```python
from build123d import *

# Parameters (mm, degrees)
SALIENTE_EXTRUIR1_DEPTH = 50.8
CROQUIS2_R              = 6.5
CORTAR_EXTRUIR1_DEPTH   = 10
CROQUIS3_R              = 6.5
CORTAR_EXTRUIR2_DEPTH   = 10
CROQUIS4_W              = 50.8
CROQUIS4_H              = 74.5
CORTAR_EXTRUIR3_DEPTH   = 10
CROQUIS5_R              = 6.35
CORTAR_EXTRUIR4_DEPTH   = 10


with BuildPart() as part:
    # Croquis1 → Saliente-Extruir1 (new body)
    with BuildSketch(Plane(origin=(0, 0, 0), x_dir=(0, 0, -1), z_dir=(1, 0, 0))):
        Polygon((-6.31, 95.93), (0, 95.93), (0, 0), (-902.2, 0), (-902.2, 6.31), (-6.31, 6.31), align=None)
    extrude(amount=SALIENTE_EXTRUIR1_DEPTH)

    # Croquis2 → Cortar-Extruir1 (cut)
    with BuildSketch(Plane(origin=(0, 0, 0), x_dir=(-1, 0, 0), z_dir=(0, -1, 0))):
        with Locations(Location((-25.4, -885.7, 0), (0, 0, 90))):
            Circle(CROQUIS2_R)
        with Locations(Location((-25.4, -854.7, 0), (0, 0, 90))):
            Circle(CROQUIS2_R)
    extrude(amount=-CORTAR_EXTRUIR1_DEPTH, mode=Mode.SUBTRACT)

    # Croquis3 → Cortar-Extruir2 (cut)
    with BuildSketch(Plane(origin=(0, 0, 0), x_dir=(-1, 0, 0), z_dir=(0, 0, -1))):
        with Locations(Location((-25.4, 70.53, 0), (0, 0, 90))):
            Circle(CROQUIS3_R)
    extrude(amount=-CORTAR_EXTRUIR2_DEPTH, mode=Mode.SUBTRACT)

    # Croquis4 → Cortar-Extruir3 (cut)
    with BuildSketch(Plane.XZ):
        with Locations((25.4, 864.95)):
            Rectangle(CROQUIS4_W, CROQUIS4_H)
    extrude(amount=-CORTAR_EXTRUIR3_DEPTH, mode=Mode.SUBTRACT)

    # Croquis5 → Cortar-Extruir4 (cut)
    with BuildSketch(Plane(origin=(0, 0, 0), x_dir=(-1, 0, 0), z_dir=(0, -1, 0))):
        with Locations(Location((-25.4, -765.81, 0), (0, 0, 90))):
            Circle(CROQUIS5_R)
        with Locations(Location((-25.4, -805.81, 0), (0, 0, 90))):
            Circle(CROQUIS5_R)
    extrude(amount=-CORTAR_EXTRUIR4_DEPTH, mode=Mode.SUBTRACT)


solid = part.part
```
Input: part model. Units: mm. Frame: model coordinates. A direction names the side the tool comes from. Give positions to 0.01 mm unless a question says otherwise; leave off trailing zeros. Order: outer loops, then holes, each group sorted by start corner. A loop starts at its lowest first (then second) coordinate and runs counter-clockwise, first axis right, second up. Notation, with made-up numbers: M 30,-28 L 68,-28 A20 cw 68,-11 Z; hole C 37,56.25 d1. An arc over 180 degrees is marked long. One line per question, with ' | ' between items. Start each with the question number.
1. Material intervals for probe 1 along X at (y, z) = (1, 805); probe 2 along X at (y, z) = (70.53, 1.5); probe 3 along Z at (x, y) = (20.5, 18.5), sorted ascending. Write a range as [from, to].
2. Pull-direction query (Y, two-part tool) for faces 1 (the face through (25, 0, 408)), 2 (the face through (25.679, 3.111, 772.154)), 3 (the face through (21.445, 65.372, 3.111)); classes: released by +Y, released by -Y, zero draft, split by the parting line, or undercut.
3. Section query A-A (x = 41). Return the cut outline in (y, z), and give its area (3 significant figures).
4. First-contact query: pin 1 Ø15 at (x, y) = (27, 55) entering from +Z; pin 2 Ø15 at (x, z) = (36.5, 469) entering from +Y; pin 3 Ø5 at (x, y) = (13.5, 14.5) entering from -Z. Flat tips, straight axial feed; report the tip coordinate or a pass-through.
5. Access query for faces 4 (the face through (25, 49, 0)), 5 (the face through (25, 50, 6.31)). Directions: +Z, -Z, +X, -X, +Y, -Y. A direction counts if a zero-diameter tool reaches every point of the face in a straight line with its end or side. Return the directions, or none.
6. Section query B-B (z = 252). Return the cut outline in (x, y), and give its area (3 significant figures).
Here are the results:
1) probe 1: [0, 19.1], [31.7, 50.8] | probe 2: [0, 18.9], [31.9, 50.8] | probe 3: [0, 6.31]
2) face 1: released by -Y | face 2: zero draft | face 3: undercut
3) outline: M 0,0 L 95.93,0 L 95.93,6.31 L 6.31,6.31 L 6.31,827.7 L 0,827.7 Z | area: 5,790 mm²
4) pin 1: z = 6.31 | pin 2: y = 6.31 | pin 3: z = 0
5) face 4: -Z, +X, -X, +Y, -Y | face 5: +Z, +X, -X, +Y
6) outline: M 0,0 L 50.8,0 L 50.8,6.31 L 0,6.31 Z | area: 321 mm²
